The model under review builds one solid part; all positions refer to its coordinate system, in mm. A direction names the side the tool comes from. Give positions to 0.01 mm unless a question says otherwise; leave off trailing zeros. Order: outer loops, then holes, each group sorted by start corner. A loop starts at its lowest first (then second) coordinate and runs counter-clockwise, first axis right, second up. Notation, with made-up numbers: (52, 78.25) - (109, 78.25) arc R30 cw to (109, 112.25) - close; hole circle Ø2 at (59, 2.25). An arc over 180 degrees is marked (long way). Put each result on its own line as item: value.
```python
from build123d import *

# Parameters (mm, degrees)
SKETCH1_W                 = 14.8
SKETCH1_H                 = 15
BOSS_EXTRUDE1_DEPTH       = 8.2
SKETCH3_W                 = 8.8
SKETCH3_H                 = 5.2
CUT_EXTRUDE1_DEPTH        = 12
SKETCH5_W                 = 10.8
SKETCH5_H                 = 1.7
CUT_EXTRUDE2_DEPTH        = 12
SKETCH6_W                 = 14.8
SKETCH6_H                 = 3
BOSS_EXTRUDE2_DEPTH       = 26
SKETCH7_R                 = 5
CUT_EXTRUDE3_DEPTH        = 36.273928049
M3X0_5_TAPPED_HOLE1_D     = 2.5
M3X0_5_TAPPED_HOLE1_DEPTH = 7.5
M3X0_5_TAPPED_HOLE1_TIP   = 0.751075774
FILLET1_R                 = 3


with BuildPart() as part:
    # Sketch1 → Boss-Extrude1 (new body)
    with BuildSketch(Plane(origin=(0, 0, 0), x_dir=(1, 0, 0), z_dir=(0, 1, 0))):
        Rectangle(SKETCH1_W, SKETCH1_H)
    extrude(amount=BOSS_EXTRUDE1_DEPTH)

    # Sketch3 → Cut-Extrude1 (cut)
    with BuildSketch(Plane.XY.offset(7.5)):
        with Locations((0, 2.6)):
            Rectangle(SKETCH3_W, SKETCH3_H)
    extrude(amount=-CUT_EXTRUDE1_DEPTH, mode=Mode.SUBTRACT)

    # Sketch5 → Cut-Extrude2 (cut)
    with BuildSketch(Plane.XY.offset(7.5)):
        with Locations((0, 2.35)):
            Rectangle(SKETCH5_W, SKETCH5_H)
    extrude(amount=-CUT_EXTRUDE2_DEPTH, mode=Mode.SUBTRACT)

    # Sketch6 → Boss-Extrude2 (add)
    with BuildSketch(Plane(origin=(0, 0, -7.5), x_dir=(-1, 0, 0), z_dir=(0, 0, -1))):
        with Locations((0, 6.7)):
            Rectangle(SKETCH6_W, SKETCH6_H)
    extrude(amount=BOSS_EXTRUDE2_DEPTH)

    # Sketch7 → Cut-Extrude3 (cut, through all)
    with BuildSketch(Plane(origin=(0, 8.2, 0), x_dir=(1, 0, 0), z_dir=(0, 1, 0))):
        with Locations(Location((0, 17.5, 0), (0, 0, 270))):
            Circle(SKETCH7_R)
    extrude(amount=-CUT_EXTRUDE3_DEPTH, mode=Mode.SUBTRACT)

    # M3x0.5 Tapped Hole1
    with Locations(Plane(origin=(0, 8.2, 0), x_dir=(1, 0, 0), z_dir=(0, 1, 0))):
        with Locations((0, 29.5)):
            Hole(M3X0_5_TAPPED_HOLE1_D / 2, depth=M3X0_5_TAPPED_HOLE1_DEPTH)
            with Locations((0, 0, -(M3X0_5_TAPPED_HOLE1_DEPTH + M3X0_5_TAPPED_HOLE1_TIP / 2))):  # 118° drill point
                Cone(0, M3X0_5_TAPPED_HOLE1_D / 2, M3X0_5_TAPPED_HOLE1_TIP, mode=Mode.SUBTRACT)

    # Fillet1
    fillet1_edges = [part.edges().sort_by_distance(p)[0] for p in [
        (0, 5.2, -7.5),
    ]]
    fillet(fillet1_edges, radius=FILLET1_R)


solid = part.part
```
(1) Take a section at C-C, the plane y = 6. Write out the cut boundary in (x, z), then the cut area to 3 significant figures.
The answers:
outline: (-7.4, -33.5) - (7.4, -33.5) - (7.4, 7.5) - (-7.4, 7.5) - close; hole circle Ø10 at (0, -17.5); hole circle Ø2.5 at (0, -29.5)
area: 523 mm^2
(2) Clearance check with flat-ended pins moving along their axes: pin 1 Ø2.5 at (x, y) = (-2, 3) entering from +Z; pin 2 Ø1.8 at (x, y) = (2, 0.5) entering from -Z; pin 3 Ø7.5 at (x, z) = (-1, -19) entering from -Y; pin 4 Ø2 at (x, z) = (0, -29.5) entering from -Y. State where each tip first meets the part, or that it passes through.
The answers:
pin 1: z = -4.5
pin 2: z = -7.5
pin 3: y = 5.2
pin 4: through
(3) Take a section at B-B, the plane x = 3. Write out the cut boundary in (y, z), then the cut area to 3 significant figures.
The answers:
outline: (0, -7.5) - (2.2, -7.5) arc R3 cw to (5.2, -10.5) - (5.2, -13.5) - (8.2, -13.5) - (8.2, 7.5) - (5.2, 7.5) - (5.2, -4.5) - (0, -4.5) - close; (5.2, -33.5) - (8.2, -33.5) - (8.2, -21.5) - (5.2, -21.5) - close
area: 117 mm^2
(4) Take a section at D-D, the plane z = 2. Write out the cut boundary in (x, y).
The answers:
outline: (-7.4, 0) - (-4.4, 0) - (-4.4, 1.5) - (-5.4, 1.5) - (-5.4, 3.2) - (-4.4, 3.2) - (-4.4, 5.2) - (4.4, 5.2) - (4.4, 3.2) - (5.4, 3.2) - (5.4, 1.5) - (4.4, 1.5) - (4.4, 0) - (7.4, 0) - (7.4, 8.2) - (-7.4, 8.2) - close
(5) The part is to be moulded in two halves that separate along Y. For faces 6 (the cylindrical face through (0.27, 6.68, -28.28)), 7 (the flat face through (0, 5.2, 2)), 8 (the flat face through (5, 3.2, 2)), say which applies: pulls with the +Y half, pulls with the -Y half, needs draft (parallel to the pull), parting line crosses it, or undercut.
The answers:
face 6: needs draft
face 7: pulls with the -Y half
face 8: undercut
(6) For faces 1 (the flat face through (-7.4, 5, -8)), 2 (the flat face through (4.4, 4, 2)), 3 (the flat face through (5, 1.5, 2)), 4 (the cylindrical face through (0.22, 6.721, -22.495)), 5 (the flat face through (0, 1, -7.5)), list the 3-axis set-ups (+Z, -Z, +X, -X, +Y, -Y) from which the entire face can be reached by the end or side of a thin tool; tool diameter is ignored.
The answers:
face 1: +Z, -Z, -X, +Y, -Y
face 2: +Z, -Y
face 3: +Z
face 4: +Y, -Y
face 5: -Z, +X, -X, -Y
(7) Wall thickness on L1, parallel to X at y = 7, z = -29.5; L2, parallel to X at y = 6.7, z = -17.5; L3, parallel to Z at x = 0.75, y = 5.5: over which ranges is each line inside the solid? List them lowest first.
The answers:
L1: -7.4 to -1.25, 1.25 to 7.4
L2: -7.4 to -5, 5 to 7.4
L3: -33.5 to -30.5, -28.5 to -22.44, -12.56 to 7.5
(8) Take a section at A-A, the plane z = -20.5. Write out the cut boundary in (x, y), then the cut area to 3 significant figures.
The answers:
outline: (-7.4, 5.2) - (-4, 5.2) - (-4, 8.2) - (-7.4, 8.2) - close; (4, 5.2) - (7.4, 5.2) - (7.4, 8.2) - (4, 8.2) - close
area: 20.4 mm^2
